Part model, mm, in its own coordinate system. Face numbers are marked on the shaded views. Give positions to 0.01 mm unless a question says otherwise; leave off trailing zeros. Write each loop counter-clockwise with the first axis right and the second up, starting at its lowest first coordinate (ties: lowest second). Pieces come first, ordered by that corner, then holes. Notation, with made-up numbers: M 83.5,-22.5 L 140.5,-22.5 A20 ccw 140.5,-9.5 Z; hole C -7,-4 d8. An arc over 180 degrees is marked long. Use CSV: the item, a comma, the result in double quotes. Start each with the question number.
Item 1: Cut at C-C (z = 33.5). List the corners of the cut face in (x, y).
Item 2: Cut at D-D (y = 2.5). List the corners of the cut face in (x, z).
Item 3: Pin check, flat tips, straight feed: pin 1 (6 mm diameter, centred on x = -31, y = 1.5, fed in from -Z); pin 2 (4 mm diameter, centred on y = 3, z = 16, fed in from -X); pin 3 (2.5 mm diameter, centred on x = 22.5, y = -2, fed in from +Z). Stop position of each tip, or through.
Item 4: Drill centre lines: line 1 (Z direction, x = 0, y = 3.55); line 2 (Z direction, x = 5.5, y = 0.25); line 3 (X direction, y = 4.75, z = 13). Where is each one in solid material? Low to high. Write a range as [from, to].
Item 5: Cut at A-A (z = -42). List the corners of the cut face in (x, y), then the cut area to 3 significant figures.
Item 6: Mould opens along Z. For the marked faces 1 and 2 say: released by +Z, released by -Z, zero draft, split by the parting line, or undercut.
Item 7: Cut at B-B (x = 36.5). List the corners of the cut face in (y, z), then the cut area to 3 significant figures.
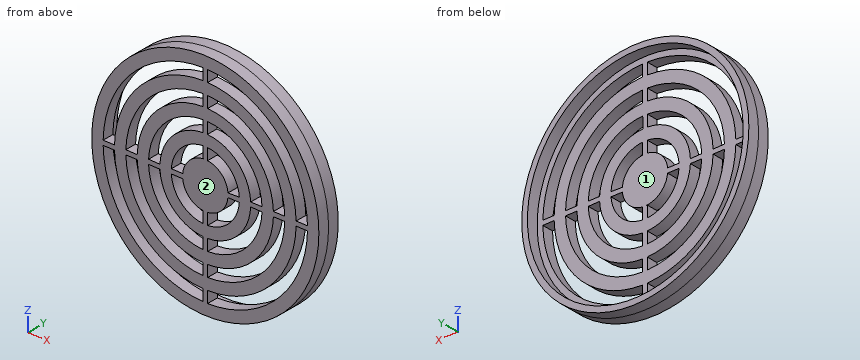
from build123d import *

# Parameters (mm, degrees)
F0_R      = 50
F1_DEPTH  = 5
F3_DEPTH  = 25
F5_DEPTH  = 25
F7_DEPTH  = 25
F9_DEPTH  = 25
F10_R     = 50
F10_R_2   = 47.5
F11_DEPTH = 5


with BuildPart() as f1:
    # F0 (on Front) → F1 (new body)
    with BuildSketch(Plane.XZ):
        Circle(F0_R)
    extrude(amount=F1_DEPTH)

    # F2 (on face) → F3 (cut)
    with BuildSketch(Plane.XZ.offset(5)):
        with BuildLine():
            Line((39.98749959, 0.9999382697), (44.9888888889, 0.9999382697))
            ThreePointArc((44.9888888889, 0.9999382697), (31.8198051534, 31.8198051534), (0.9999382697, 44.9888888889))
            Line((0.9999382697, 44.9888888889), (0.9999382697, 39.98749959))
            ThreePointArc((0.9999382697, 39.98749959), (28.2842712475, 28.2842712475), (39.98749959, 0.9999382697))
        make_face()
        with BuildLine():
            ThreePointArc((0.9999382697, -44.9888888889), (31.8198051534, -31.8198051534), (44.9888888889, -0.9999382697))
            Line((44.9888888889, -0.9999382697), (39.9888503033, -0.9443788557))
            ThreePointArc((39.9888503033, -0.9443788557), (28.3039134456, -28.2646153992), (0.9999382697, -39.98749959))
            Line((0.9999382697, -39.98749959), (0.9999382697, -44.9888888889))
        make_face()
        with BuildLine():
            Line((-0.9999382697, 39.98749959), (-0.9999382697, 44.9888888889))
            ThreePointArc((-0.9999382697, 44.9888888889), (-31.8198051534, 31.8198051534), (-44.9888888889, 0.9999382697))
            Line((-44.9888888889, 0.9999382697), (-39.98749959, 0.9999382697))
            ThreePointArc((-39.98749959, 0.9999382697), (-28.2842712475, 28.2842712475), (-0.9999382697, 39.98749959))
        make_face()
        with BuildLine():
            ThreePointArc((-44.9888888889, -0.9999382697), (-31.8198051534, -31.8198051534), (-0.9999382697, -44.9888888889))
            Line((-0.9999382697, -44.9888888889), (-0.9999382697, -39.98749959))
            ThreePointArc((-0.9999382697, -39.98749959), (-28.2842712475, -28.2842712475), (-39.98749959, -0.9999382697))
            Line((-39.98749959, -0.9999382697), (-44.9888888889, -0.9999382697))
        make_face()
    extrude(amount=-F3_DEPTH, mode=Mode.SUBTRACT)

    # F4 (on face) → F5 (cut)
    with BuildSketch(Plane.XZ.offset(5)):
        with BuildLine():
            Line((-0.999897954, 29.9833321044), (-0.999897954, 34.9857142857))
            ThreePointArc((-0.999897954, 34.9857142857), (-24.7487373415, 24.7487373415), (-34.9857142857, 0.999897954))
            Line((-34.9857142857, 0.999897954), (-29.9856292313, 0.9284608776))
            ThreePointArc((-29.9856292313, 0.9284608776), (-21.2384582595, 21.1879185094), (-0.999897954, 29.9833321044))
        make_face()
        with BuildLine():
            Line((-29.9833321044, -0.999897954), (-34.9857142857, -0.999897954))
            ThreePointArc((-34.9857142857, -0.999897954), (-24.7487373415, -24.7487373415), (-0.999897954, -34.9857142857))
            Line((-0.999897954, -34.9857142857), (-0.999897954, -29.9833321044))
            ThreePointArc((-0.999897954, -29.9833321044), (-21.2132034356, -21.2132034356), (-29.9833321044, -0.999897954))
        make_face()
        with BuildLine():
            ThreePointArc((0.999897954, -34.9857142857), (24.7487373415, -24.7487373415), (34.9857142857, -0.999897954))
            Line((34.9857142857, -0.999897954), (29.9833321044, -0.999897954))
            ThreePointArc((29.9833321044, -0.999897954), (21.2132034356, -21.2132034356), (0.999897954, -29.9833321044))
            Line((0.999897954, -29.9833321044), (0.999897954, -34.9857142857))
        make_face()
        with BuildLine():
            ThreePointArc((34.9857131335, 0.9999382697), (24.7487230819, 24.7487516011), (0.999897954, 34.9857142857))
            Line((0.999897954, 34.9857142857), (0.999897954, 29.9833321044))
            ThreePointArc((0.999897954, 29.9833321044), (21.2131891739, 21.2132176973), (29.9833307599, 0.9999382697))
            Line((29.9833307599, 0.9999382697), (34.9857131335, 0.9999382697))
        make_face()
    extrude(amount=-F5_DEPTH, mode=Mode.SUBTRACT)

    # F6 (on face) → F7 (cut)
    with BuildSketch(Plane(origin=(0, 0, 0), x_dir=(-1, 0, 0), z_dir=(0, 1, 0))):
        with BuildLine():
            Line((19.9797498734, 0.8997749705), (24.98, 0.99979998))
            ThreePointArc((24.98, 0.99979998), (17.6776695297, 17.6776695297), (0.99979998, 24.98))
            Line((0.99979998, 24.98), (0.99979998, 19.974994368))
            ThreePointArc((0.99979998, 19.974994368), (14.1774954339, 14.106687181), (19.9797498734, 0.8997749705))
        make_face()
        with BuildLine():
            ThreePointArc((0.99979998, -24.98), (17.6776695297, -17.6776695297), (24.98, -0.99979998))
            Line((24.98, -0.99979998), (19.974994368, -0.99979998))
            ThreePointArc((19.974994368, -0.99979998), (14.1421356237, -14.1421356237), (0.99979998, -19.974994368))
            Line((0.99979998, -19.974994368), (0.99979998, -24.98))
        make_face()
        with BuildLine():
            ThreePointArc((-24.98, -0.99979998), (-17.6776695297, -17.6776695297), (-0.99979998, -24.98))
            Line((-0.99979998, -24.98), (-0.99979998, -19.974994368))
            ThreePointArc((-0.99979998, -19.974994368), (-14.1774954339, -14.106687181), (-19.9797498734, -0.8997749705))
            Line((-19.9797498734, -0.8997749705), (-24.98, -0.99979998))
        make_face()
        with BuildLine():
            Line((-0.8997749705, 19.9797498734), (-0.99979998, 24.98))
            ThreePointArc((-0.99979998, 24.98), (-17.6776695297, 17.6776695297), (-24.98, 0.99979998))
            Line((-24.98, 0.99979998), (-19.974994368, 0.99979998))
            ThreePointArc((-19.974994368, 0.99979998), (-14.106687181, 14.1774954339), (-0.8997749705, 19.9797498734))
        make_face()
    extrude(amount=-F7_DEPTH, mode=Mode.SUBTRACT)

    # F8 (on face) → F9 (cut)
    with BuildSketch(Plane.XZ.offset(5)):
        with BuildLine():
            Line((-0.99944429, 10), (-0.99944429, 14.9666666667))
            ThreePointArc((-0.99944429, 14.9666666667), (-10.6066017178, 10.6066017178), (-14.9666666667, 0.99944429))
            Line((-14.9666666667, 0.99944429), (-9.9499302063, 0.99944429))
            ThreePointArc((-9.9499302063, 0.99944429), (-6.8917841678, 7.2459168492), (-0.5000354957, 9.9874904006))
            Line((-0.5000354957, 9.9874904006), (-0.99944429, 10))
        make_face()
        with BuildLine():
            Line((10, 0.8337966825), (14.9666666667, 0.99944429))
            ThreePointArc((14.9666666667, 0.99944429), (10.6066017178, 10.6066017178), (0.99944429, 14.9666666667))
            Line((0.99944429, 14.9666666667), (0.99944429, 9.9499302063))
            ThreePointArc((0.99944429, 9.9499302063), (7.2614861704, 6.8753777058), (9.989650171, 0.4548510314))
            Line((9.989650171, 0.4548510314), (10, 0.8337966825))
        make_face()
        with BuildLine():
            ThreePointArc((0.99944429, -14.9666666667), (10.6066017178, -10.6066017178), (14.9666666667, -0.99944429))
            Line((14.9666666667, -0.99944429), (9.9499302063, -0.99944429))
            ThreePointArc((9.9499302063, -0.99944429), (7.0710678119, -7.0710678119), (0.99944429, -9.9499302063))
            Line((0.99944429, -9.9499302063), (0.99944429, -14.9666666667))
        make_face()
        with BuildLine():
            ThreePointArc((-14.9666666667, -0.99944429), (-10.6066017178, -10.6066017178), (-0.99944429, -14.9666666667))
            Line((-0.99944429, -14.9666666667), (-0.99944429, -10))
            Line((-0.99944429, -10), (-0.5000354957, -9.9874904006))
            ThreePointArc((-0.5000354957, -9.9874904006), (-6.8917841678, -7.2459168492), (-9.9499302063, -0.99944429))
            Line((-9.9499302063, -0.99944429), (-14.9666666667, -0.99944429))
        make_face()
    extrude(amount=-F9_DEPTH, mode=Mode.SUBTRACT)

    # F10 (on face) → F11 (join)
    with BuildSketch(Plane(origin=(0, 0, 0), x_dir=(-1, 0, 0), z_dir=(0, 1, 0))):
        Circle(F10_R)
        Circle(F10_R_2, mode=Mode.SUBTRACT)
    extrude(amount=F11_DEPTH)


solid = f1.part
Worked answers:
1,outline,"M -37.12,-5 L -30.05,-5 L -30.05,0 L -33.67,0 L -33.67,5 L -37.12,5 Z; M -21.86,-5 L -10.14,-5 L -10.14,0 L -21.86,0 Z; M -1,-5 L 1,-5 L 1,0 L -1,0 Z; M 10.14,-5 L 21.86,-5 L 21.86,0 L 10.14,0 Z; M 30.05,-5 L 37.12,-5 L 37.12,5 L 33.67,5 L 33.67,0 L 30.05,0 Z"
2,outline,"C 0,0 d100; hole C 0,0 d95"
3,pin 1,"stops at z = -41.42"
3,pin 2,"stops at x = -48"
3,pin 3,"stops at z = 45.26"
4,line 1,"z = [-50, -47.5], [47.5, 50]"
4,line 2,"z = [-49.7, -47.18], [47.18, 49.7]"
4,line 3,"x = [-48.28, -45.69], [45.69, 48.28]"
5,outline,"M -27.13,-5 L -16.16,-5 L -16.16,0 L -22.19,0 L -22.19,5 L -27.13,5 Z; M -1,-5 L 1,-5 L 1,0 L -1,0 Z; M 16.16,-5 L 27.13,-5 L 27.13,5 L 22.19,5 L 22.19,0 L 16.16,0 Z"
5,area,"169 mm^2"
6,face 1,"undercut"
6,face 2,"zero draft"
7,outline,"M -5,-34.17 L 5,-34.17 L 5,-30.4 L 0,-30.4 L 0,-26.32 L -5,-26.32 Z; M -5,-16.36 L 0,-16.36 L 0,16.36 L -5,16.36 Z; M -5,26.32 L 0,26.32 L 0,30.4 L 5,30.4 L 5,34.17 L -5,34.17 Z"
7,area,"280 mm^2"
